```python
from build123d import *

# Parameters (mm, degrees)
SKETCH2_R                            = 10
SKETCH2_R_2                          = 1.65
BOSS_EXTRUDE1_DEPTH                  = 6.35
CUT_EXTRUDE1_DEPTH                   = 10
FILLET3_R                            = 3
SKETCH5_R                            = 1.75
CUT_EXTRUDE2_DEPTH                   = 549.511460792
SKETCH6_R                            = 26.5
CUT_EXTRUDE3_DEPTH                   = 10
BOSS_EXTRUDE2_START                  = -6.35
BOSS_EXTRUDE2_DEPTH                  = 6.35
TAP_DRILL_FOR_M3X0_5_TAP1_AT_2_COUNT = 2
TAP_DRILL_FOR_M3X0_5_TAP1_AT_2_PITCH = 12
CIRPATTERN2_COUNT                    = 2
CIRPATTERN2_ANGLE                    = 90
CUT_EXTRUDE4_DEPTH                   = 549.511460792
SKETCH11_R                           = 36
CUT_EXTRUDE5_DEPTH                   = 549.511460792
CUT_EXTRUDE6_DEPTH                   = 549.511460792
CUT_EXTRUDE6_DEPTH_BACK              = 549.511460792
SKETCH12_R                           = 1.25


with BuildPart() as part:
    # Sketch2 → Boss-Extrude1 (new body)
    with BuildSketch(Plane.XY):
        with BuildLine():
            Line((-46.5, 0), (-46.5, 500))
            ThreePointArc((-46.5, 500), (0, 546.5), (46.5, 500))
            Line((46.5, 500), (46.5, 0))
            ThreePointArc((46.5, 0), (0, -46.5), (-46.5, 0))
        make_face()
        Circle(SKETCH2_R, mode=Mode.SUBTRACT)
        with Locations((0, 13.75)):
            Circle(SKETCH2_R_2, mode=Mode.SUBTRACT)
        with Locations((11.907849302, 6.875)):
            Circle(SKETCH2_R_2, mode=Mode.SUBTRACT)
        with Locations((11.907849302, -6.875)):
            Circle(SKETCH2_R_2, mode=Mode.SUBTRACT)
        with Locations((0, -13.75)):
            Circle(SKETCH2_R_2, mode=Mode.SUBTRACT)
        with Locations((-11.907849302, -6.875)):
            Circle(SKETCH2_R_2, mode=Mode.SUBTRACT)
        with Locations((-11.907849302, 6.875)):
            Circle(SKETCH2_R_2, mode=Mode.SUBTRACT)
    extrude(amount=BOSS_EXTRUDE1_DEPTH)

    # Sketch4 → Cut-Extrude1 (cut)
    with BuildSketch(Plane.XY.offset(6.35)):
        Polygon((28.005258112, 59.37595418), (0, 42.411661153), (-28.005258112, 59.37595418), (0, 141.693437584), align=None)
        Polygon((-7.5, 156.905935087), (-28.005258112, 96.633637735), (-28.005258112, 167.582877854), align=None)
        Polygon((28.005258112, 167.582877854), (7.5, 156.905935087), (28.005258112, 96.633637735), align=None)
        with BuildLine():
            Line((0, 164.275138905), (28.550546746, 179.141206521))
            add(Edge.make_bspline(
                [(28.550546746, 179.141206521), (45.32025339, 216.985654627), (19.430092874, 259.790255689), (0, 290.025756679)],
                knots=[0, 0, 0, 0, 1, 1, 1, 1], degree=3))
            add(Edge.make_bspline(
                [(-28.550546746, 179.141206521), (-45.32025339, 216.985654627), (-19.430092874, 259.790255689), (0, 290.025756679)],
                knots=[0, 0, 0, 0, 1, 1, 1, 1], degree=3))
            Line((-28.550546746, 179.141206521), (0, 164.275138905))
        make_face()
        Polygon((28.550546746, 259.58677623), (3, 314.938284003), (28.550546746, 340.793051053), align=None)
        Polygon((-3, 314.938284003), (-28.550546746, 340.793051053), (-28.550546746, 259.58677623), align=None)
        Polygon((0, 423.142843498), (-28.550546746, 369.246205395), (0, 340.355718526), (28.550546746, 369.246205395), align=None)
        Polygon((-28.550546746, 462.095190817), (-28.550546746, 401.290241252), (-11, 434.421497018), align=None)
        Polygon((28.550546746, 401.290241252), (11, 434.421497018), (28.550546746, 462.095190817), align=None)
    extrude(amount=-CUT_EXTRUDE1_DEPTH, mode=Mode.SUBTRACT)

    # Fillet3
    fillet3_edges = [part.edges().sort_by_distance(p)[0] for p in [
        (-11, 434.421497018, 3.175),
        (-28.550546746, 401.290241252, 3.175),
        (28.550546746, 401.290241252, 3.175),
        (11, 434.421497018, 3.175),
        (28.550546746, 462.095190817, 3.175),
        (-28.550546746, 462.095190817, 3.175),
        (0, 423.142843498, 3.175),
        (-28.550546746, 369.246205395, 3.175),
        (28.550546746, 369.246205395, 3.175),
        (0, 340.355718526, 3.175),
        (28.550546746, 340.793051053, 3.175),
        (-28.550546746, 340.793051053, 3.175),
        (-3, 314.938284003, 3.175),
        (3, 314.938284003, 3.175),
        (28.550546746, 259.58677623, 3.175),
        (-28.550546746, 259.58677623, 3.175),
        (28.550546746, 179.141206521, 3.175),
        (0, 290.025756679, 3.175),
        (-28.550546746, 179.141206521, 3.175),
        (0, 164.275138905, 3.175),
        (-28.005258112, 96.633637735, 3.175),
        (28.005258112, 96.633637735, 3.175),
        (7.5, 156.905935087, 3.175),
        (-28.005258112, 167.582877854, 3.175),
        (28.005258112, 167.582877854, 3.175),
        (0, 141.693437584, 3.175),
        (28.005258112, 59.37595418, 3.175),
        (-28.005258112, 59.37595418, 3.175),
        (0, 42.411661153, 3.175),
        (-7.5, 156.905935087, 3.175),
    ]]
    fillet(fillet3_edges, radius=FILLET3_R)

    # Sketch5 → Cut-Extrude2 (cut, through all)
    with BuildSketch(Plane.XY.offset(6.35)):
        with Locations((36.5, 103.175)):
            Circle(SKETCH5_R)
        with Locations(Location((-36.5, 103.175, 0), (0, 0, 180))):
            Circle(SKETCH5_R)
        with Locations(Location((36.5, 259.525, 0), (0, 0, 180))):
            Circle(SKETCH5_R)
        with Locations((-36.5, 259.525)):
            Circle(SKETCH5_R)
        with Locations((36.5, 415.875)):
            Circle(SKETCH5_R)
        with Locations(Location((-36.5, 415.875, 0), (0, 0, 180))):
            Circle(SKETCH5_R)
    extrude(amount=-CUT_EXTRUDE2_DEPTH, mode=Mode.SUBTRACT)

    # Sketch6 → Cut-Extrude3 (cut)
    with BuildSketch(Plane.XY.offset(6.35)):
        with Locations((0, 500)):
            Circle(SKETCH6_R)
    extrude(amount=-CUT_EXTRUDE3_DEPTH, mode=Mode.SUBTRACT)

    # Sketch7 → Boss-Extrude2 (add)
    with BuildSketch(Plane.XY.offset(6.35).offset(BOSS_EXTRUDE2_START)):
        with BuildLine():
            Line((44.110383395, 529.968247771), (29.968247771, 544.110383395))
            ThreePointArc((29.968247771, 544.110383395), (23.286397782, 542.399293624), (16.474718596, 543.483717035))
            ThreePointArc((16.474718596, 543.483717035), (32.880465325, 532.880465325), (43.483717035, 516.474718596))
            ThreePointArc((43.483717035, 516.474718596), (42.399293624, 523.286397782), (44.110383395, 529.968247771))
        make_face()
    boss_extrude2 = extrude(amount=BOSS_EXTRUDE2_DEPTH)

    # Sketch9 → Tap Drill for M3x0.5 Tap1 (revolve, cut)
    with BuildSketch(Plane(origin=(32.796674896, 541.28195627, 3.175), x_dir=(-0.7071067811865481, 0.7071067811865469, 0), z_dir=(0, 0, 1))):
        Polygon((0, 0), (0, 5.751075774), (1.25, 5), (1.25, 0), align=None)
    tap_drill_for_m3x0_5_tap1 = revolve(axis=Axis((37.286802956, 545.772084331, 3.175), (-0.7071067811865468, -0.7071067811865482, 0)), mode=Mode.SUBTRACT)

    # Tap Drill for M3x0.5 Tap1 at 2: Tap Drill for M3x0.5 Tap1 ×2
    with Locations(*[Vector(0.7071067811865482, -0.7071067811865468, 0) * (i * TAP_DRILL_FOR_M3X0_5_TAP1_AT_2_PITCH) for i in range(1, TAP_DRILL_FOR_M3X0_5_TAP1_AT_2_COUNT)]):
        add(tap_drill_for_m3x0_5_tap1, mode=Mode.SUBTRACT)

    # CirPattern2: Boss-Extrude2, Tap Drill for M3x0.5 Tap1 ×2 about axis
    cirpattern2_axis = Axis((0, 500, 0), (0, 0, 1))
    add([boss_extrude2.rotate(cirpattern2_axis, i * CIRPATTERN2_ANGLE / (CIRPATTERN2_COUNT - 1)) for i in range(1, CIRPATTERN2_COUNT)])
    add([tap_drill_for_m3x0_5_tap1.rotate(cirpattern2_axis, i * CIRPATTERN2_ANGLE / (CIRPATTERN2_COUNT - 1)) for i in range(1, CIRPATTERN2_COUNT)], mode=Mode.SUBTRACT)

    # CirPattern2 copy 1 sketch → CirPattern2 copy 1 (revolve, cut)
    with BuildSketch(Plane(origin=(-32.796674896, 541.28195627, 3.175), x_dir=(-0.7071067811865445, -0.7071067811865506, 0), z_dir=(0, 0, 1))):
        Polygon((0, 0), (0, 5.751075774), (1.25, 5), (1.25, 0), align=None)
    revolve(axis=Axis((-37.286802956, 545.772084331, 3.175), (0.7071067811865507, -0.7071067811865444, 0)), mode=Mode.SUBTRACT)

    # Sketch10 → Cut-Extrude4 (cut, through all)
    with BuildSketch(Plane.XY.offset(6.35)):
        with BuildLine():
            Line((-43.483717035, 516.474718596), (-63.483717035, 516.474718596))
            ThreePointArc((-63.483717035, 516.474718596), (0, 565.586573942), (63.483717035, 516.474718596))
            Line((63.483717035, 516.474718596), (43.483717035, 516.474718596))
            ThreePointArc((43.483717035, 516.474718596), (0, 546.5), (-43.483717035, 516.474718596))
        make_face()
    extrude(amount=-CUT_EXTRUDE4_DEPTH, mode=Mode.SUBTRACT)

    # Sketch11 → Cut-Extrude5 (cut, through all)
    with BuildSketch(Plane.XY.offset(6.35)):
        with Locations((0, 500)):
            Circle(SKETCH11_R)
    extrude(amount=-CUT_EXTRUDE5_DEPTH, mode=Mode.SUBTRACT)

    # Sketch12 → Cut-Extrude6 (cut, two sides: drawn at the far end of the back side and taken through both)
    with BuildSketch(Plane.XY.offset(6.35).offset(-CUT_EXTRUDE6_DEPTH_BACK)):
        with Locations((0, 541.25)):
            Circle(SKETCH12_R)
        with Locations((20.625, 535.723547906)):
            Circle(SKETCH12_R)
        with Locations((35.723547906, 520.625)):
            Circle(SKETCH12_R)
        with Locations((41.25, 500)):
            Circle(SKETCH12_R)
        with Locations((35.723547906, 479.375)):
            Circle(SKETCH12_R)
        with Locations((20.625, 464.276452094)):
            Circle(SKETCH12_R)
        with Locations((0, 458.75)):
            Circle(SKETCH12_R)
        with Locations((-20.625, 464.276452094)):
            Circle(SKETCH12_R)
        with Locations((-35.723547906, 479.375)):
            Circle(SKETCH12_R)
        with Locations((-41.25, 500)):
            Circle(SKETCH12_R)
        with Locations((-35.723547906, 520.625)):
            Circle(SKETCH12_R)
        with Locations((-20.625, 535.723547906)):
            Circle(SKETCH12_R)
    extrude(amount=CUT_EXTRUDE6_DEPTH + CUT_EXTRUDE6_DEPTH_BACK, mode=Mode.SUBTRACT)


solid = part.part
```
Input: part model. Units: mm. Frame: model coordinates. Coordinates: 2 decimals unless noted, no trailing zeros. Write each loop counter-clockwise with the first axis right and the second up, starting at its lowest first coordinate (ties: lowest second). Pieces come first, ordered by that corner, then holes.
1) Pin query (flat end, axial travel): pin 1 Ø2 at (x, y) = (-35.72, 479.38) entering from +Z; pin 2 Ø1 at (x, z) = (-12.5, 5.5) entering from +Y; pin 3 Ø1.5 at (x, z) = (-36, 3.5) entering from -Y. Return the tip coordinate at first contact, or that it passes through.
2) Section B-B on z = 2.75. State how many separate pieces and enclosed holes the cut face has, and give its area (3 significant figures).
3) Mould query, pull axis Y, two halves, no side actions, for faces 1 (the flat face through (21.3, 254.2, 0)), 2 (the flat face through (-17.4, 444.51, 3.22)), 3 (the flat face through (17.4, 444.51, 3.22)). Classes: pulls with the +Y half, pulls with the -Y half, needs draft (parallel to the pull), parting line crosses it, or undercut.
4) Material intervals for line 1 along X through (y, z) = (153.5, 5.25); line 2 along Y through (x, z) = (2.5, 1.75); line 3 along X through (y, z) = (321.5, 1), sorted ascending.
5) Section A-A on y = 142. Output: boundary loops of the cut face in (x, z).
Check result:
1. pin 1: passes through
1. pin 2: stops at y = 544.92
1. pin 3: stops at y = -30.33
2. separate pieces: 1
2. enclosed holes: 35
2. area: 33,500 mm2
3. face 1: needs draft
3. face 2: undercut
3. face 3: undercut
4. line 1: x = -46.5 to -28.01, -8.66 to 8.66, 28.01 to 46.5
4. line 2: y = -46.43 to -9.68, 9.68 to 43.93, 134.04 to 165.58, 286.12 to 342.89, 418.39 to 464.09, 535.91 to 546.43
4. line 3: x = -46.5 to -28.55, -9.48 to 9.48, 28.55 to 46.5
5. outline: (-46.5, 0) - (-28.01, 0) - (-28.01, 6.35) - (-46.5, 6.35) - close; (-12.57, 0) - (12.57, 0) - (12.57, 6.35) - (-12.57, 6.35) - close; (28.01, 0) - (46.5, 0) - (46.5, 6.35) - (28.01, 6.35) - close
